Autodesk Inventor part; units mm, degrees
ref_plane "YZ Plane" through (0, 0, 0) normal (1, 0, 0) x (0, 1, 0)
ref_plane "XZ Plane" through (0, 0, 0) normal (0, 1, 0) x (-1, 0, 0)
ref_plane "XY Plane" through (0, 0, 0) normal (0, 0, 1) x (1, 0, 0)
sketch "Sketch1" plane through (0, 0, 0) normal (0, 0, 1) x (1, 0, 0)
  line L0 (-12.1708, 16.0073) -> (13.2292, 16.0073)
  line L1 (13.2292, 16.0073) -> (13.2292, -34.7927)
  line L2 (13.2292, -34.7927) -> (-12.1708, -34.7927)
  line L3 (-12.1708, -34.7927) -> (-12.1708, 16.0073)
  line L4 (11.9592, 14.7373) -> (-10.9008, 14.7373)
  line L5 (-10.9008, 14.7373) -> (-10.9008, -33.5227)
  line L6 (-10.9008, -33.5227) -> (11.9592, -33.5227)
  line L7 (11.9592, -33.5227) -> (11.9592, 14.7373)
  point P0 (0, 0)
  dimension "d0" = 25.4
  dimension "d1" = 50.8
  dimension "d2" = 1.27
extrude "Extrusion1" add sketch "Sketch1" along normal blind 111.76
sketch "Sketch2" plane through (-12.1708, 16.0073, 0) normal (0, 1, 0) x (1, 0, 0)
  circle A0 centre (12.7, -12.7) radius 1.7272
  line L0 (25.4, 0) -> (0, 0)
  line L1 (0, 0) -> (0, -111.76)
  point P0 (12.1708, 0)
  dimension "d5" = 3.4544
  dimension "d6" = 12.7
  dimension "d7" = 12.7
extrude "Extrusion2" cut sketch "Sketch2" against normal through all
pattern_linear "Rectangular Pattern1" count 11 spacing 25.4 along (0, 0, 1) of "Extrusion2"
sketch "Sketch3" plane through (13.2292, -34.7927, 0) normal (1, 0, 0) x (0, 0, -1)
  circle A0 centre (-60.96, 25.4) radius 14.2875
  line L0 (0, 0) -> (-111.76, 0)
  line L1 (-111.76, 0) -> (-111.76, 50.8)
  point P0 (0, 34.7927)
  dimension "d15" = 25.4
  dimension "d16" = 50.8
  dimension "d17" = 28.575
extrude "Extrusion3" cut sketch "Sketch3" against normal through all
equation "\"d3\" = d13"
equation "\"d10\" = d14"
equation "\"d13\" = 111.76"
equation "\"d14\" = d13"
properties part number "Test  Stock Rotation extender"
Source: CAD feature listing. Evaluate the final solid. Frame: model axes, mm. A direction names the side the tool comes from. Coordinates: 2 decimals unless noted, no trailing zeros. Order: outer loops, then holes, each group sorted by start corner. A loop starts at its lowest first (then second) coordinate and runs counter-clockwise, first axis right, second up. Notation, with made-up numbers: M 42.25,-37.5 L 98.25,-37.5 A22 cw 98.25,-29.5 Z; hole C -25,51.5 d9. An arc over 180 degrees is marked long. Write each question's results on one line, items separated by ' | '. Start each with the question number.
1) Line query: line 1 (Y direction, x = -0.75, z = 34); line 2 (X direction, y = 2.5, z = 104.5); line 3 (Y direction, x = 12.85, z = 60.96). Output: solid intervals per line, ascending. Write a range as from..to.
2) Section query D-D (z = 29.5). Return the cut outline in (x, y).
3) Draft query along Z for faces 3 (the face through (-12, -9, 111.76)), 4 (the face through (1, -34.793, 55)), 5 (the face through (12.603, -18.086, 72.298)). Return one class per face: released by +Z, released by -Z, zero draft, split by the parting line, or undercut.
4) Section query B-B (x = 8). Return the cut outline in (y, z), plus the area to 3 significant figures.
5) Section query C-C (y = -7.5). Return the cut outline in (x, z).
6) Contact query for a flat-ended pin moving along its axis: pin 1 Ø3 at (x, z) = (0.53, 63.5) entering from +Y. Output: stop coordinate, or through.
7) Access query for faces 1 (the face through (11.959, -10, 43)), 2 (the face through (0.3, -34.15, 87.19)). Directions: +Z, -Z, +X, -X, +Y, -Y. A direction counts if a zero-diameter tool reaches every point of the face in a straight line with its end or side. Return the directions, or none.
8) Section query A-A (z = 12.7). Return the cut outline in (x, y), plus the area to 3 significant figures.
Answers:
1) line 1: y = -34.79..-33.52, 14.74..16.01 | line 2: x = -12.17..-10.9, 11.96..13.23 | line 3: y = -34.79..-23.68, 4.89..16.01
2) outline: M -12.17,-34.79 L 13.23,-34.79 L 13.23,16.01 L -12.17,16.01 Z; hole M -10.9,-33.52 L 11.96,-33.52 L 11.96,14.74 L -10.9,14.74 Z
3) face 3: released by +Z | face 4: zero draft | face 5: undercut
4) outline: M -34.79,0 L -33.52,0 L -33.52,111.76 L -34.79,111.76 Z; M 14.74,0 L 16.01,0 L 16.01,111.76 L 14.74,111.76 Z | area: 284 mm^2
5) outline: M -12.17,0 L -10.9,0 L -10.9,46.8 L -12.17,46.8 Z; M -12.17,75.12 L -10.9,75.12 L -10.9,111.76 L -12.17,111.76 Z; M 11.96,0 L 13.23,0 L 13.23,46.8 L 11.96,46.8 Z; M 11.96,75.12 L 13.23,75.12 L 13.23,111.76 L 11.96,111.76 Z
6) pin 1: passes through
7) face 1: +Z, -Z | face 2: +Y, -Y
8) outline: M -12.17,-34.79 L -1.2,-34.79 L -1.2,-33.52 L -10.9,-33.52 L -10.9,14.74 L -1.2,14.74 L -1.2,16.01 L -12.17,16.01 Z; M 2.26,-34.79 L 13.23,-34.79 L 13.23,16.01 L 2.26,16.01 L 2.26,14.74 L 11.96,14.74 L 11.96,-33.52 L 2.26,-33.52 Z | area: 178 mm^2
